Part model, mm, in its own coordinate system. A direction names the side the tool comes from. Give positions to 0.01 mm unless a question says otherwise; leave off trailing zeros. Order: outer loops, then holes, each group sorted by start corner. A loop starts at its lowest first (then second) coordinate and runs counter-clockwise, first axis right, second up. Notation, with made-up numbers: (44.5, 82) -> (83.5, 82) arc R11 ccw to (83.5, 87) -> close; hole circle Ø4 at (3, -4). An arc over 180 degrees is marked (long way). Write item = value, one per line. Start each with the question number.
(1) Two-plate mould, pull along Y, no slides. Class faces 6 (the flat face through (25, 31, 10)), 7 (the flat face through (14, 20, 10)), 8 (the flat face through (40.732, 6.628, 16.056)): pulls with the +Y half, pulls with the -Y half, needs draft (parallel to the pull), parting line crosses it, or undercut.
(2) Saw through at A-A, the plane z = 18.25. List the corners of the cut face in (x, y).
(3) Saw through at C-C, the plane y = 4.5. List the corners of the cut face in (x, z).
(4) Which spindle directions (+Z, -Z, +X, -X, +Y, -Y) get a long thin tool onto all of the face, cutting with end or side? Do faces 1 (the flat face through (45, 31, 10)), 2 (the flat face through (25, -11, 10)), 3 (the flat face through (35, 18, 0)), 4 (the flat face through (29.268, 13.372, 16.056)), 5 (the flat face through (45, -11, 10)). Say none if no direction does.
(5) Saw through at D-D, the plane x = 20. List the corners of the cut face in (y, z).
(6) Probe line 1 along Y through (x, z) = (35, 10.25); line 2 along Y through (x, z) = (62.5, 15.5); line 3 along X through (y, z) = (21, 12). List the from-to ranges inside material, lowest first. Write a range as from..to.
(7) Flat gauge pins, fed straight in: pin 1 (10 mm diameter, centred on x = 60, z = 7, fed in from -Y); pin 2 (6 mm diameter, centred on x = 50.5, z = 10.5, fed in from +Y); pin 3 (10 mm diameter, centred on y = 25.5, z = 10, fed in from +X). Where does each tip first touch, or does it go through?
(8) Saw through at B-B, the plane x = 35. List the corners of the cut face in (y, z).
from build123d import *

# Parameters (mm, degrees)
ESQUISSE1_W             = 20
ESQUISSE1_H             = 25
ESQUISSE1_H_2           = 20
ESQUISSE1_W_2           = 25
BOSS_EXTRU_1_DEPTH      = 20
ENL_V_MAT_EXTRU_1_REACH = 87.586
ESQUISSE2_R             = 4.05
ENL_V_MAT_EXTRU_3_DEPTH = 8
CONG_1_R                = 3


with BuildPart() as part:
    # Esquisse1 → Boss.-Extru.1 (new body)
    with BuildSketch(Plane.XY):
        with Locations((35, 32.5)):
            Rectangle(ESQUISSE1_W, ESQUISSE1_H)
        with Locations((35, 10)):
            Rectangle(ESQUISSE1_W, ESQUISSE1_H_2)
        with Locations((12.5, 10)):
            Rectangle(ESQUISSE1_W_2, ESQUISSE1_H_2)
        with Locations((35, -12.5)):
            Rectangle(ESQUISSE1_W, ESQUISSE1_H)
        with Locations((57.5, 10)):
            Rectangle(ESQUISSE1_W_2, ESQUISSE1_H_2)
    extrude(amount=BOSS_EXTRU_1_DEPTH)

    # Esquisse2 → Enlèv. mat.-Extru.1 (cut, up to next)
    with BuildSketch(Plane.XY.offset(20), mode=Mode.PRIVATE) as enl_v_mat_extru_1_sk1:
        with Locations((35, 10)):
            Circle(ESQUISSE2_R)
    enl_v_mat_extru_1_tool1 = extrude(enl_v_mat_extru_1_sk1.sketch, amount=-ENL_V_MAT_EXTRU_1_REACH, mode=Mode.PRIVATE) & part.part
    add(enl_v_mat_extru_1_tool1.solids().sort_by_distance((35, 10, 20))[0], mode=Mode.SUBTRACT)

    # Esquisse4 → Enlèv. mat.-Extru.3 (cut)
    with BuildSketch(Plane.XY.offset(20)):
        Polygon((27.32124142, 10), (31.16062071, 3.35), (38.83937929, 3.35), (42.67875858, 10), (38.83937929, 16.65), (31.16062071, 16.65), align=None)
    extrude(amount=-ENL_V_MAT_EXTRU_3_DEPTH, mode=Mode.SUBTRACT)

    # Congé1
    cong_1_edges = [part.edges().sort_by_distance(p)[0] for p in [
        (45, 45, 10),
        (70, 20, 10),
        (70, 0, 10),
        (45, -25, 10),
        (25, -25, 10),
        (0, 0, 10),
        (0, 20, 10),
        (25, 45, 10),
    ]]
    fillet(cong_1_edges, radius=CONG_1_R)


solid = part.part
Results list:
q1.face_6 = needs draft
q1.face_7 = pulls with the +Y half
q1.face_8 = undercut
q2.outline = (0, 3) arc R3 ccw to (3, 0) -> (25, 0) -> (25, -22) arc R3 ccw to (28, -25) -> (42, -25) arc R3 ccw to (45, -22) -> (45, 0) -> (67, 0) arc R3 ccw to (70, 3) -> (70, 17) arc R3 ccw to (67, 20) -> (45, 20) -> (45, 42) arc R3 ccw to (42, 45) -> (28, 45) arc R3 ccw to (25, 42) -> (25, 20) -> (3, 20) arc R3 ccw to (0, 17) -> close; hole (27.32, 10) -> (31.16, 3.35) -> (38.84, 3.35) -> (42.68, 10) -> (38.84, 16.65) -> (31.16, 16.65) -> close
q3.outline = (0, 0) -> (70, 0) -> (70, 20) -> (39.5, 20) -> (39.5, 12) -> (30.5, 12) -> (30.5, 20) -> (0, 20) -> close
q4.face_1 = +Z, -Z, +X, +Y
q4.face_2 = +Z, -Z, -X, -Y
q4.face_3 = -Z, +X, -X, +Y, -Y
q4.face_4 = +Z
q4.face_5 = +Z, -Z, +X, -Y
q5.outline = (0, 0) -> (20, 0) -> (20, 20) -> (0, 20) -> close
q6.line_1 = -25..5.95, 14.05..45
q6.line_2 = 0..20
q6.line_3 = 25..45
q7.pin_1 = 0
q7.pin_2 = 20
q7.pin_3 = 45
q8.outline = (-25, 0) -> (5.95, 0) -> (5.95, 12) -> (3.35, 12) -> (3.35, 20) -> (-25, 20) -> close; (14.05, 0) -> (45, 0) -> (45, 20) -> (16.65, 20) -> (16.65, 12) -> (14.05, 12) -> close
